```python
from build123d import *

# Parameters (mm, degrees)
SKETCH1_R                 = 9.94
SKETCH1_R_2               = 7.94
BOSS_EXTRUDE3_DEPTH       = 5
SKETCH1_6_R               = 7.94
SKETCH1_6_R_2             = 4.94
BOSS_EXTRUDE4_DEPTH       = 18
BOSS_EXTRUDE7_DEPTH       = 40
BOSS_EXTRUDE7_DEPTH_BACK  = 70
SKETCH4_R                 = 25
SKETCH4_R_2               = 23
SKETCH7_W                 = 197.712308018
SKETCH7_H                 = 113.854833504
CUT_EXTRUDE4_DEPTH        = 64
BOSS_EXTRUDE9_START       = -2
SKETCH9_RX                = 35.355339059
SKETCH9_RY                = 25
SKETCH9_R                 = 4.94
BOSS_EXTRUDE9_DEPTH       = 2
SKETCH13_W                = 94.503894001
SKETCH13_H                = 33.113273172
CUT_EXTRUDE7_DEPTH        = 32
BOSS_EXTRUDE11_START      = -2
BOSS_EXTRUDE11_DEPTH      = 2
BOSS_EXTRUDE12_DEPTH      = 2
BOSS_EXTRUDE12_DEPTH_BACK = 4


with BuildPart() as part:
    # Sketch1 → Boss-Extrude3 (new body)
    with BuildSketch(Plane(origin=(0, 0, 0), x_dir=(1, 0, 0), z_dir=(0, 1, 0))):
        with Locations(Location((0, 0, 0), (0, 0, 270))):
            Circle(SKETCH1_R)
        with Locations(Location((0, 0, 0), (0, 0, 270))):
            Circle(SKETCH1_R_2, mode=Mode.SUBTRACT)
    extrude(amount=BOSS_EXTRUDE3_DEPTH)

    # Sketch1<6> → Boss-Extrude4 (add)
    with BuildSketch(Plane(origin=(0, 0, 0), x_dir=(1, 0, 0), z_dir=(0, 1, 0))):
        with Locations(Location((0, 0, 0), (0, 0, 270))):
            Circle(SKETCH1_6_R)
        with Locations(Location((0, 0, 0), (0, 0, 270))):
            Circle(SKETCH1_6_R_2, mode=Mode.SUBTRACT)
    extrude(amount=BOSS_EXTRUDE4_DEPTH)



with BuildPart() as body_2:
    # Sketch4 → Boss-Extrude7 (new, two sides: drawn at the far end of the back side and taken through both)
    with BuildSketch(Plane(origin=(0, -5.365491749, 5.365491749), x_dir=(-1, 0, 0), z_dir=(0, 0.7071067811865458, -0.7071067811865492)).offset(-BOSS_EXTRUDE7_DEPTH_BACK)):
        with Locations(Location((0, 0, 0), (0, 0, 90))):
            Circle(SKETCH4_R)
        with Locations(Location((0, 0, 0), (0, 0, 90))):
            Circle(SKETCH4_R_2, mode=Mode.SUBTRACT)
    extrude(amount=BOSS_EXTRUDE7_DEPTH + BOSS_EXTRUDE7_DEPTH_BACK)

    # Sketch7 → Cut-Extrude4 (cut)
    with BuildSketch(Plane(origin=(0, 0, 0), x_dir=(1, 0, 0), z_dir=(0, 1, 0))):
        Rectangle(SKETCH7_W, SKETCH7_H)
    extrude(amount=CUT_EXTRUDE4_DEPTH, mode=Mode.SUBTRACT)


with BuildPart() as part_1:
    add(part.part)

    add(body_2.part)  # Boss-Extrude9 merges body 2
    # Sketch9 → Boss-Extrude9 (add)
    with BuildSketch(Plane(origin=(0, 0, 0), x_dir=(1, 0, 0), z_dir=(0, 1, 0)).offset(BOSS_EXTRUDE9_START)):
        with Locations(Location((0, 0), (0, 0, -90))):
            Ellipse(SKETCH9_RX, SKETCH9_RY)
        with Locations(Location((0, 0, 0), (0, 0, 270))):
            Circle(SKETCH9_R, mode=Mode.SUBTRACT)
    extrude(amount=BOSS_EXTRUDE9_DEPTH)

    # Sketch13 → Cut-Extrude7 (cut)
    with BuildSketch(Plane(origin=(0, 8.776643875, -8.776643875), x_dir=(-1, 0, 0), z_dir=(0, 0.7071067811865458, -0.7071067811865492))):
        with Locations((18.042265065, -27.160500048)):
            Rectangle(SKETCH13_W, SKETCH13_H)
    extrude(amount=CUT_EXTRUDE7_DEPTH, mode=Mode.SUBTRACT)

    # Boss-Extrude11: read off the stored shape, not the designer's step
    # Boss-Extrude11 outline → Boss-Extrude11 (add)
    with BuildSketch(Plane(origin=(0, 8.776643875, -8.776643875), x_dir=(-1, 0, 0), z_dir=(0, 0.7071067811865458, -0.7071067811865492)).offset(BOSS_EXTRUDE11_START)):
        with BuildLine():
            Line((18.806642372, -13.240475924), (-18.806642372, -13.240475924))
            ThreePointArc((-18.806642372, -13.240475924), (0, -23), (18.806642372, -13.240475924))
        make_face()
    extrude(amount=BOSS_EXTRUDE11_DEPTH)

    # Sketch15 → Boss-Extrude12 (add, two sides: drawn at the far end of the back side and taken through both)
    with BuildSketch(Plane(origin=(0, -13, 0), x_dir=(1, 0, 0), z_dir=(0, 1, 0)).offset(-BOSS_EXTRUDE12_DEPTH_BACK)):
        Polygon((-18, 50.5), (-18, 5.077623205), (-11, 12.425207431), (0.436295729, 16.20866498), (9.681434559, 13.33514052), (16.664877802, 7.136081647), (20.985766733, 0), (38, 24.667240496), (38, 50.5), (31, 50.5), (31, 26.250403727), (-11, 26.250403727), (-11, 50.5), align=None)
    extrude(amount=BOSS_EXTRUDE12_DEPTH + BOSS_EXTRUDE12_DEPTH_BACK)


solid = part_1.part
```
CAD build for the part. Positions are in the model's coordinates, mm. A direction names the side the tool comes from. Round coordinates to 2 decimals unless told otherwise and drop trailing zeros. Order: outer loops, then holes, each group sorted by start corner. A loop starts at its lowest first (then second) coordinate and runs counter-clockwise, first axis right, second up. Notation, with made-up numbers: (4, 45.5) - (37, 45.5) arc R18 ccw to (37, 70.5) - close; hole circle Ø5 at (39, 22). An arc over 180 degrees is marked (long way). Answer in a Markdown table with one row per item. Add a question column.
(1) Drop flat-ended pins along their axis: pin 1 Ø5 at (y, z) = (-15, -37.5) entering from -X; pin 2 Ø2 at (y, z) = (-13.5, -7) entering from -X; pin 3 Ø2 at (y, z) = (-34, 21.5) entering from -X; pin 4 Ø6 at (x, z) = (-3, 1) entering from +Y. Give the stop position or say it passes through.
(2) Band-saw the part on A-A on x = 29.5. List the corners of the cut face in (y, z).
(3) Probe L1, parallel to X at y = 5.5, z = 0; L2, parallel to X at y = 4, z = 0; L3, parallel to Z at x = 2, y = -7. List the from-to ranges inside material, lowest first. Write a range as [from, to].
(4) Mould opens along Z. For faces 4 (the face through (-7.291, -39.232, 70.494)), 5 (the face through (-14.55, -13.81, -8.7)), 6 (the face through (-18, -14, -29)) say: +Z half, -Z half, draft (parallel to the pull), parting line (faces both ways), or undercut.
(5) 3-axis set-ups, long thin cutter, end or side, ignore diameter. For faces 1 (the face through (-11, -14, -38)), 2 (the face through (-23, -2, -13)), 3 (the face through (2, -11, -16)): which of +Z, -Z, +X, -X, +Y, -Y reach the whole face in a straight line?
Data:
| question | item | result |
|---|---|---|
| 1 | pin 1 | stops at x = -18 |
| 1 | pin 2 | stops at x = -21.04 |
| 1 | pin 3 | stops at x = -23.74 |
| 1 | pin 4 | stops at y = 18 |
| 2 | outline | (-17, -26.25) - (-11, -26.25) - (-11, -12.34) - (-17, -12.34) - close |
| 3 | L1 | x = [-7.94, -4.94], [4.94, 7.94] |
| 3 | L2 | x = [-9.94, -4.94], [4.94, 9.94] |
| 3 | L3 | z = [-24.55, -21.72], [39.4, 42.24] |
| 4 | face 4 | +Z half |
| 4 | face 5 | undercut |
| 4 | face 6 | draft |
| 5 | face 1 | -Z, +Y, -Y |
| 5 | face 2 | -Z, -X, -Y |
| 5 | face 3 | none |
